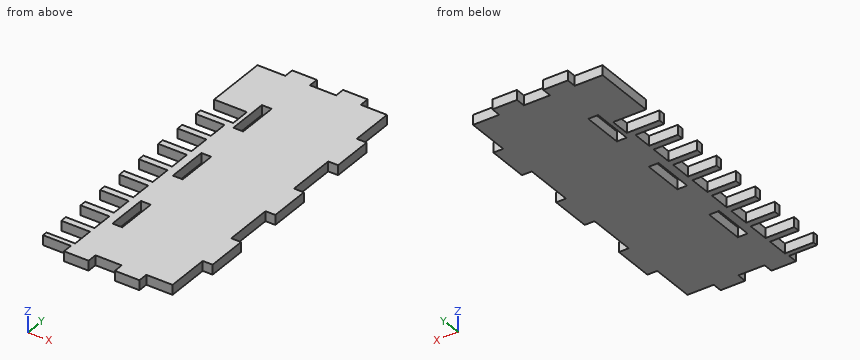
from build123d import *

# Parameters (mm, degrees)
ESQUISSE1_W             = 79
ESQUISSE1_H             = 188
BOSS_EXTRU_1_DEPTH      = 6
ESQUISSE2_W             = 20
ESQUISSE2_H             = 12
ESQUISSE2_W_2           = 17.5
ESQUISSE2_H_2           = 13
ENL_V_MAT_EXTRU_1_DEPTH = 10
ESQUISSE3_W             = 6
ESQUISSE3_H             = 25
BOSS_EXTRU_2_DEPTH      = 6
ESQUISSE4_W             = 15
ESQUISSE4_H             = 6
BOSS_EXTRU_3_DEPTH      = 6
ESQUISSE5_W             = 15
ESQUISSE5_H             = 6
BOSS_EXTRU_4_DEPTH      = 6
ESQUISSE6_W             = 6
ESQUISSE6_H             = 25
ESQUISSE6_W_2           = 5.984999771
ESQUISSE6_W_3           = 6.000000529
ENL_V_MAT_EXTRU_2_DEPTH = 10


with BuildPart() as part:
    # Esquisse1 → Boss.-Extru.1 (new body)
    with BuildSketch(Plane.XY):
        Rectangle(ESQUISSE1_W, ESQUISSE1_H)
    extrude(amount=BOSS_EXTRU_1_DEPTH)

    # Esquisse2 → Enlèv. mat.-Extru.1 (cut)
    with BuildSketch(Plane.XY.offset(6)):
        with Locations((-29.5, 50)):
            Rectangle(ESQUISSE2_W, ESQUISSE2_H)
        with Locations((-30.75, 34)):
            Rectangle(ESQUISSE2_W_2, ESQUISSE2_H)
        with Locations((-30.75, 17.5)):
            Rectangle(ESQUISSE2_W_2, ESQUISSE2_H_2)
        with Locations((-30.75, 0.5)):
            Rectangle(ESQUISSE2_W_2, ESQUISSE2_H_2)
        with Locations((-30.75, -16.5)):
            Rectangle(ESQUISSE2_W_2, ESQUISSE2_H_2)
        with Locations((-30.75, -33.5)):
            Rectangle(ESQUISSE2_W_2, ESQUISSE2_H_2)
        with Locations((-30.75, -50.5)):
            Rectangle(ESQUISSE2_W_2, ESQUISSE2_H_2)
        with Locations((-30.75, -67.5)):
            Rectangle(ESQUISSE2_W_2, ESQUISSE2_H_2)
        with Locations((-30.75, -84.5)):
            Rectangle(ESQUISSE2_W_2, ESQUISSE2_H_2)
    extrude(amount=-ENL_V_MAT_EXTRU_1_DEPTH, mode=Mode.SUBTRACT)

    # Esquisse3 → Boss.-Extru.2 (add)
    with BuildSketch(Plane(origin=(39.5, 0, 0), x_dir=(0, 0, -1), z_dir=(1, 0, 0))):
        with Locations((-3, 55)):
            Rectangle(ESQUISSE3_W, ESQUISSE3_H)
        with Locations((-3, 0)):
            Rectangle(ESQUISSE3_W, ESQUISSE3_H)
        with Locations((-3, -55)):
            Rectangle(ESQUISSE3_W, ESQUISSE3_H)
    extrude(amount=BOSS_EXTRU_2_DEPTH)

    # Esquisse4 → Boss.-Extru.3 (add)
    with BuildSketch(Plane(origin=(0, 94, 0), x_dir=(1, 0, 0), z_dir=(0, 1, 0))):
        with Locations((-15, -3)):
            Rectangle(ESQUISSE4_W, ESQUISSE4_H)
        with Locations((16, -3)):
            Rectangle(ESQUISSE4_W, ESQUISSE4_H)
    extrude(amount=BOSS_EXTRU_3_DEPTH)

    # Esquisse5 → Boss.-Extru.4 (add)
    with BuildSketch(Plane.XZ.offset(94)):
        with Locations((16, 3)):
            Rectangle(ESQUISSE5_W, ESQUISSE5_H)
        with Locations((-15, 3)):
            Rectangle(ESQUISSE5_W, ESQUISSE5_H)
    extrude(amount=BOSS_EXTRU_4_DEPTH)

    # Esquisse6 → Enlèv. mat.-Extru.2 (cut)
    with BuildSketch(Plane(origin=(0, 0, 0), x_dir=(-1, 0, 0), z_dir=(0, 0, -1))):
        with Locations((14, -53)):
            Rectangle(ESQUISSE6_W, ESQUISSE6_H)
        with Locations((14.007500115, -4.018e-06)):
            Rectangle(ESQUISSE6_W_2, ESQUISSE6_H)
        with Locations((13.999999736, 52.999991964)):
            Rectangle(ESQUISSE6_W_3, ESQUISSE6_H)
    extrude(amount=-ENL_V_MAT_EXTRU_2_DEPTH, mode=Mode.SUBTRACT)


solid = part.part
CAD build for the part. Positions are in the model's coordinates, mm. Round coordinates to 2 decimals unless told otherwise and drop trailing zeros. Write each loop counter-clockwise with the first axis right and the second up, starting at its lowest first coordinate (ties: lowest second). Pieces come first, ordered by that corner, then holes. Notation, with made-up numbers: M 81.5,-19.75 L 97.5,-19.75 A23 ccw 97.5,10.25 Z; hole C 49,47.5 d4. An arc over 180 degrees is marked long. Put each result on its own line as item: value. Start each with the question number.
1) Saw through at C-C, the plane y = 14.5. Write the cut outline in (x, z).
2) Saw through at A-A, the plane y = -59. Write the cut outline in (x, z), and give its area (3 significant figures).
3) Saw through at D-D, the plane z = 1.5. Count the separate pieces of the cut face and the enclosed holes in it, and give its area (3 significant figures).
4) Drill centre lines: probe 1 along Y at (x, z) = (41, 1.05); probe 2 along Y at (x, z) = (-15.5, 2.15); probe 3 along X at (y, z) = (83, 0.4). Where is each one in solid material? Low to high. Write a range as [from, to].
5) Saw through at B-B, the plane x = 28. Write the cut outline in (y, z), and give its area (3 significant figures).
6) Pin check, flat tips, straight feed: pin 1 Ø1.8 at (x, z) = (-28, 3.5) entering from -Y; pin 2 Ø1 at (x, z) = (-26.5, 1) entering from +Y; pin 3 Ø5 at (x, y) = (-1, -1.5) entering from -Z; pin 4 Ø3 at (x, z) = (44, 3.5) entering from +Y. Stop position of each tip, or through.
Resolved:
1. outline: M -22,0 L 39.5,0 L 39.5,6 L -22,6 Z
2. outline: M -39.5,0 L -17,0 L -17,6 L -39.5,6 Z; M -11,0 L 45.5,0 L 45.5,6 L -11,6 Z
2. area: 474 mm²
3. separate pieces: 1
3. enclosed holes: 3
3. area: 13,200 mm²
4. probe 1: [-67.5, -42.5], [-12.5, 12.5], [42.5, 67.5]
4. probe 2: [-100, -65.5], [-40.5, -12.5], [12.5, 40.5], [65.5, 100]
4. probe 3: [-39.5, 39.5]
5. outline: M -94,0 L 94,0 L 94,6 L -94,6 Z
5. area: 1,130 mm²
6. pin 1: y = -94
6. pin 2: y = 94
6. pin 3: z = 0
6. pin 4: y = 67.5
